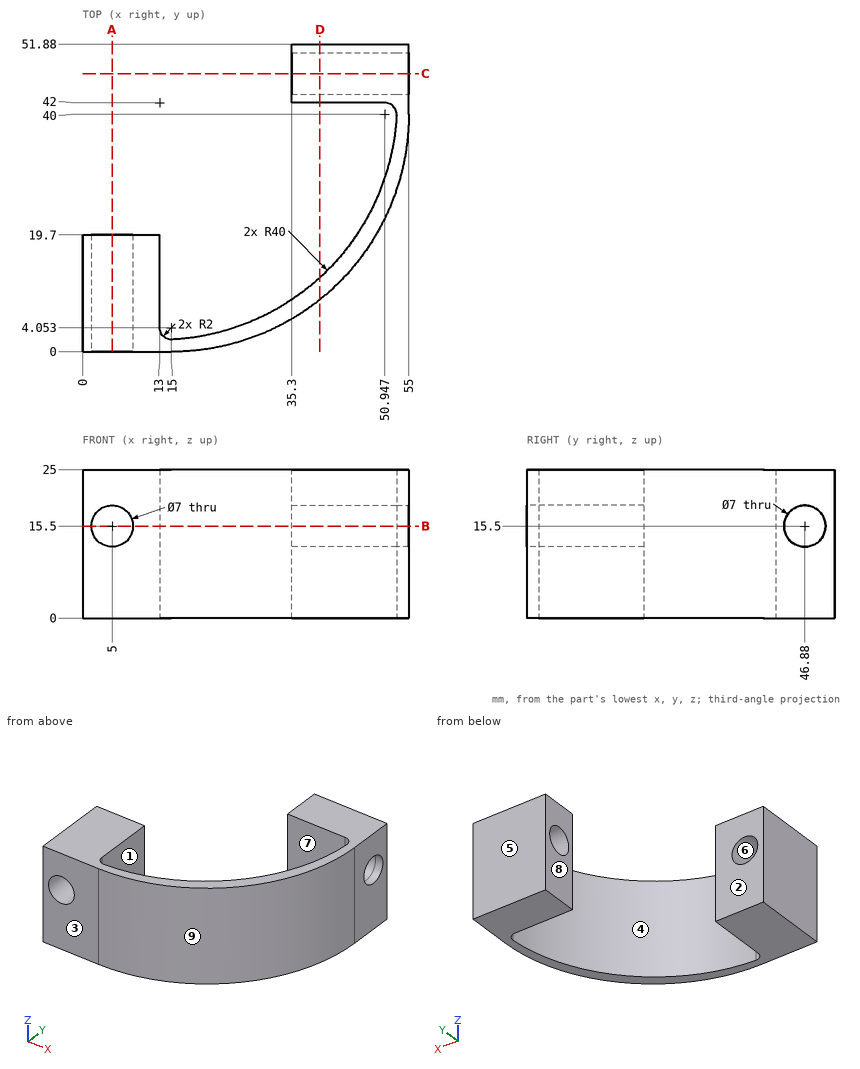
Study the drawing (mm; zero at the part's minimum x, y, z) and answer. A direction names the side the tool comes from. Coordinates: 2 decimals unless noted, no trailing zeros. Write each loop counter-clockwise with the first axis right and the second up, starting at its lowest first coordinate (ties: lowest second). Pieces come first, ordered by that corner, then holes. Notation, with made-up numbers: M -9.5,70.25 L 17.5,70.25 A20 ccw 17.5,108.25 Z; hole C -12,31.25 d5. An arc over 180 degrees is marked long. Use a Markdown table: item, result. Add a question column.
1. Section A-A (x = 5) is taken. Give the vertices of the cut face in (y, z).
2. Given P1, Ø1, axis at y = 36, z = 5.5, coming from the -X side; P2, Ø8, axis at y = 46.88, z = 15.5, coming from the -X side; P3, Ø5, axis at y = 25, z = 4, coming from the +X side; P4, Ø6.5, axis at x = 5, z = 15.5, coming from the -Y side, each flat-ended and moving along its own axis, determine where each tip first touches the part or whether it passes through.
3. Section B-B (z = 15.5) is taken. Give the vertices of the cut face in (x, y) (1 decimal), plus the area to 3 significant figures.
4. Section D-D (x = 40) is taken. Give the vertices of the cut face in (y, z) (1 decimal), plus the area to 3 significant figures.
5. Straight lines are drawn through the part: line 1 along Y through (x, z) = (41.5, 15.5) (1 decimal); line 2 along X through (y, z) = (15.75, 15.5); line 3 along X through (y, z) = (10.5, 15.5) (1 decimal). For each, find the intervals that lie inside material, in ascending order. Write a range as [from, to].
6. For a pull along X with two mould halves and no side action, classify the marked faces 6, 7, 8 and 9 as +X half, -X half, draft (parallel to the pull), parting line (faces both ways), or undercut.
7. Section C-C (y = 46.88) is taken. Give the vertices of the cut face in (x, z), plus the area to 3 significant figures.
8. Which of the six approach directions +Z, -Z, +X, -X, +Y, -Y give full straight-line access (tool end or side, diameter ignored) to the marked faces 1, 2, 3, 4 and 5?
Data:
| question | item | result |
|---|---|---|
| 1 | outline | M 0,0 L 19.7,0 L 19.7,12 L 0,12 Z; M 0,19 L 19.7,19 L 19.7,25 L 0,25 Z |
| 2 | P1 | stops at x = 52.47 |
| 2 | P2 | stops at x = 35.3 |
| 2 | P3 | stops at x = 53 |
| 2 | P4 | passes through |
| 3 | outline | M 0,0 L 1.5,0 L 1.5,19.7 L 0,19.7 Z; M 8.5,0 L 15,0 A40 ccw 55,40 L 55,43.4 L 35.3,43.4 L 35.3,42 L 50.9,42 A2 cw 52.9,39.9 A40 cw 15.1,2.1 A2 cw 13,4.1 L 13,19.7 L 8.5,19.7 Z; M 35.3,50.4 L 55,50.4 L 55,51.9 L 35.3,51.9 Z |
| 3 | area | 341 mm2 |
| 4 | outline | M 8.8,0 L 12.5,0 L 12.5,25 L 8.8,25 Z; M 42,0 L 51.9,0 L 51.9,25 L 42,25 Z; hole C 46.9,15.5 d7 |
| 4 | area | 301 mm2 |
| 5 | line 1 | y = [10, 13.9], [42, 43.4], [50.4, 51.9] |
| 5 | line 2 | x = [0, 1.5], [8.5, 13], [43.18, 46.81] |
| 5 | line 3 | x = [0, 1.5], [8.5, 13], [37.7, 42] |
| 6 | face 6 | undercut |
| 6 | face 7 | draft |
| 6 | face 8 | -X half |
| 6 | face 9 | +X half |
| 7 | outline | M 35.3,0 L 55,0 L 55,12 L 35.3,12 Z; M 35.3,19 L 55,19 L 55,25 L 35.3,25 Z |
| 7 | area | 355 mm2 |
| 8 | face 1 | +Z, -Z, +Y |
| 8 | face 2 | +Z, -Z, -X, +Y |
| 8 | face 3 | +Z, -Z, +X, -X, -Y |
| 8 | face 4 | +Z, -Z |
| 8 | face 5 | +Z, -Z, +X, -X, +Y |
